from build123d import *

# Parameters (mm, degrees)
EXTRUDE_1_DEPTH = 0.5
SKETCH_3_R      = 2.75
EXTRUDE_2_DEPTH = 1.5
SKETCH_5_R      = 1.6
EXTRUDE_3_DEPTH = 3.6
EXTRUDE_4_DEPTH = 1


with BuildPart() as part:
    # ｽｹｯﾁ2 → ﾎﾞｽ - 押し出し1 (new, symmetric)
    with BuildSketch(Plane.XY):
        Polygon((-2, 0), (2, 0), (2.5, 0.5), (2.5, 3), (-2.5, 3), (-2.5, 0.5), align=None)
    extrude(amount=EXTRUDE_1_DEPTH, both=True)

    # ｽｹｯﾁ3 → ﾎﾞｽ - 押し出し2 (add)
    with BuildSketch(Plane(origin=(0, 3, 0), x_dir=(1, 0, 0), z_dir=(0, 1, 0))):
        with Locations(Location((0, 0, 0), (0, 0, 270))):
            Circle(SKETCH_3_R)
    extrude(amount=EXTRUDE_2_DEPTH)

    # ｽｹｯﾁ5 → ﾎﾞｽ - 押し出し3 (add)
    with BuildSketch(Plane(origin=(0, 4.5, 0), x_dir=(1, 0, 0), z_dir=(0, 1, 0))):
        with Locations(Location((0, 0, 0), (0, 0, 270))):
            Circle(SKETCH_5_R)
    extrude(amount=EXTRUDE_3_DEPTH)

    # ｽｹｯﾁ6 → ﾎﾞｽ - 押し出し4 (add)
    with BuildSketch(Plane(origin=(0, 8.1, 0), x_dir=(1, 0, 0), z_dir=(0, 1, 0))):
        with BuildLine():
            Line((-1.6, -1.15), (-1.6, 1.15))
            ThreePointArc((-1.6, 1.15), (0, 2.75), (1.6, 1.15))
            Line((1.6, 1.15), (1.6, -1.15))
            ThreePointArc((1.6, -1.15), (0, -2.75), (-1.6, -1.15))
        make_face()
    extrude(amount=EXTRUDE_4_DEPTH)


solid = part.part
Verification items for the finished model (mm, model axes). A direction names the side the tool comes from. Give positions to 0.01 mm unless a question says otherwise; leave off trailing zeros. Loops run counter-clockwise (first coordinate to the right, second up) from the corner with the lowest first, then second, coordinate; pieces in that order, holes last.
1) Draft check along Y on faces 1 (the flat face through (0, 8.1, -2)), 2 (the flat face through (0, 9.1, 0)), 3 (the cylindrical face through (0.04, 8.59, 2.75)). Enter one of: pulls with the +Y half, pulls with the -Y half, needs draft (parallel to the pull), parting line crosses it, or undercut.
2) Sectioned sample at A-A, the plane z = 2.4. Enter the section's corners in (x, y).
3) Thickness scan on line 1 along Y through (x, z) = (1.4, 1.7); line 2 along Z through (x, y) = (0.4, 2.5); line 3 along X through (y, z) = (1.25, -0.1). Record the ranges inside material, lowest first.
4) Sectioned sample at B-B, the plane x = 0. Enter the section's corners in (y, z), then the cut area to 3 significant figures.
5) Sectioned sample at D-D, the plane z = 0.95. Enter the section's corners in (x, y), then the cut area to 3 significant figures.
6) Sectioned sample at C-C, the plane y = 5.25. Enter the section's corners in (x, z).
7) Set-up check for faces 4 (the cylindrical face through (-0.04, 8.59, -2.75)), 5 (the flat face through (0, 2, -0.5)), 6 (the cylindrical face through (-0.97, 6.27, -1.27)): record each of +Z, -Z, +X, -X, +Y, -Y from which the full face is reachable in a straight line by a thin tool's end or side.
8) Depth check by flat-ended pin: pin 1 Ø0.8 at (y, z) = (1.5, 0) entering from -X; pin 2 Ø1.1 at (y, z) = (1.5, 0) entering from +X; pin 3 Ø1 at (x, y) = (-1.5, 1) entering from -Z. Enter the tip coordinate at first touch or a pass-through.
Answers:
1. face 1: undercut
1. face 2: pulls with the +Y half
1. face 3: needs draft
2. outline: (-1.34, 3) - (1.34, 3) - (1.34, 4.5) - (-1.34, 4.5) - close; (-1, 8.1) - (1, 8.1) - (1, 9.1) - (-1, 9.1) - close
3. line 1: y = 3 to 4.5, 8.1 to 9.1
3. line 2: z = -0.5 to 0.5
3. line 3: x = -2.5 to 2.5
4. outline: (0, -0.5) - (3, -0.5) - (3, -2.75) - (4.5, -2.75) - (4.5, -1.6) - (8.1, -1.6) - (8.1, -2.75) - (9.1, -2.75) - (9.1, 2.75) - (8.1, 2.75) - (8.1, 1.6) - (4.5, 1.6) - (4.5, 2.75) - (3, 2.75) - (3, 0.5) - (0, 0.5) - close
4. area: 28.3 mm2
5. outline: (-2.58, 3) - (2.58, 3) - (2.58, 4.5) - (1.29, 4.5) - (1.29, 8.1) - (1.6, 8.1) - (1.6, 9.1) - (-1.6, 9.1) - (-1.6, 8.1) - (-1.29, 8.1) - (-1.29, 4.5) - (-2.58, 4.5) - close
5. area: 20.2 mm2
6. outline: circle Ø3.2 at (0, 0)
7. face 4: -Z, +Y
7. face 5: -Z, +X, -X, -Y
7. face 6: none
8. pin 1: stops at x = -2.5
8. pin 2: stops at x = 2.5
8. pin 3: stops at z = -0.5
